from build123d import *

# Parameters (mm, degrees)
F0_W           = 55
F0_H           = 30
F1_DEPTH       = 10
F2_W           = 15
F2_H           = 5
F3_DEPTH       = 10
F4_R           = 5
F6_D           = 4.2
F6_CSINK_D     = 8.96
F6_CSINK_ANGLE = 90


with BuildPart() as f1:
    # F0 (on Top) → F1 (new body)
    with BuildSketch(Plane.XY):
        with BuildLine():
            Line((29.5, 20), (-29.5, 20))
            ThreePointArc((-29.5, 20), (-31.62132, 19.12132), (-32.5, 17))
            Line((-32.5, 17), (-32.5, -17))
            ThreePointArc((-32.5, -17), (-31.62132, -19.12132), (-29.5, -20))
            Line((-29.5, -20), (29.5, -20))
            ThreePointArc((29.5, -20), (31.62132, -19.12132), (32.5, -17))
            Line((32.5, -17), (32.5, 17))
            ThreePointArc((32.5, 17), (31.62132, 19.12132), (29.5, 20))
        make_face()
        Rectangle(F0_W, F0_H, mode=Mode.SUBTRACT)
    extrude(amount=F1_DEPTH)

    # F2 (on face) → F3 (join)
    with BuildSketch(Plane.XY.offset(10)):
        with Locations((-13.75, -17.5)):
            Rectangle(F2_W, F2_H)
        with Locations((13.75, -17.5)):
            Rectangle(F2_W, F2_H)
    extrude(amount=F3_DEPTH)

    # F4
    f4_edges = [f1.edges().sort_by_distance(p)[0] for p in [
        (-21.25, -17.5, 20),
        (-6.25, -17.5, 20),
        (6.25, -17.5, 20),
        (21.25, -17.5, 20),
    ]]
    fillet(f4_edges, radius=F4_R)

    # F6 (through all)
    with Locations(Plane(origin=(0, -15, 0), x_dir=(-1, 0, 0), z_dir=(0, 1, 0))):
        with Locations((13.75, 15), (-13.75, 15)):
            CounterSinkHole(F6_D / 2, F6_CSINK_D / 2, counter_sink_angle=F6_CSINK_ANGLE)


solid = f1.part
Model file for the job. Use its own axes, mm. A direction names the side the tool comes from. Give positions to 0.01 mm unless a question says otherwise; leave off trailing zeros. Loops run counter-clockwise (first coordinate to the right, second up) from the corner with the lowest first, then second, coordinate; pieces in that order, holes last.
Item 1: Slice it at C-C (x = -25.5). Write the cut outline in (y, z), plus the area to 3 significant figures.
Check values:
outline: (-20, 0) - (-15, 0) - (-15, 10) - (-20, 10) - close; (15, 0) - (20, 0) - (20, 10) - (15, 10) - close
area: 100 mm2
Item 2: Slice it at B-B (y = 3.5). Write the cut outline in (x, z), plus the area to 3 significant figures.
Check values:
outline: (-32.5, 0) - (-27.5, 0) - (-27.5, 10) - (-32.5, 10) - close; (27.5, 0) - (32.5, 0) - (32.5, 10) - (27.5, 10) - close
area: 100 mm2
Item 3: Mould opens along Y. For faces 4 (the face through (-27.5, 0, 5)), 5 (the face through (-31.6, 19.14, 4.93)), 6 (the face through (27.5, 0, 5)), 7 (the face through (0, -20, 8)) say: +Y half, -Y half, draft (parallel to the pull), parting line (faces both ways), or undercut.
Check values:
face 4: undercut
face 5: +Y half
face 6: undercut
face 7: -Y half
Item 4: Slice it at A-A (x = -13.75). Write the cut outline in (y, z).
Check values:
outline: (-20, 0) - (-15, 0) - (-15, 10.52) - (-17.38, 12.9) - (-20, 12.9) - close; (-20, 17.1) - (-17.38, 17.1) - (-15, 19.48) - (-15, 20) - (-20, 20) - close; (15, 0) - (20, 0) - (20, 10) - (15, 10) - close
Item 5: Which spindle directions (+Z, -Z, +X, -X, +Y, -Y) get a long thin tool onto all of the face, cutting with end or side? Do faces 1 (the face through (0, 15, 5)), 2 (the face through (21.25, -18, 12)), 3 (the face through (-7.75, -17.46, 18.57)). Say none if no direction does.
Check values:
face 1: +Z, -Z
face 2: +Z, +X, +Y, -Y
face 3: +Z, +Y, -Y
Item 6: Drill centre lines: line 1 along X through (y, z) = (-18.2, 15); line 2 along Y through (x, z) = (24, 6.25); line 3 along X through (y, z) = (1.5, 8.75). Where is each one in solid material? Low to high.
Check values:
line 1: x = -21.25 to -15.85, -11.65 to -6.25, 6.25 to 11.65, 15.85 to 21.25
line 2: y = -20 to -15, 15 to 20
line 3: x = -32.5 to -27.5, 27.5 to 32.5
Item 7: Slice it at D-D (x = 15). Give the number of separate pieces and of enclosed holes in the cut face, plus the area to 3 significant figures.
Check values:
separate pieces: 3
enclosed holes: 0
area: 127 mm2
Item 8: Drop flat-ended pins along their axis: P1, Ø1.5, axis at x = 0, y = -17.5, coming from the +Z side; P2, Ø2.5, axis at y = -17, z = 12, coming from the +X side; P3, Ø2.5, axis at y = -17, z = 13, coming from the -X side. Give the stop position or say it passes through.
Check values:
P1: stops at z = 10
P2: stops at x = 21.25
P3: stops at x = -21.25
